```python
from build123d import *

# Parameters (mm, degrees)
SKETCH1_R           = 2.794
BOSS_EXTRUDE1_DEPTH = 2.54
SKETCH2_R           = 3.556
BOSS_EXTRUDE2_DEPTH = 6.35
SKETCH3_R           = 1.397
CUT_EXTRUDE1_DEPTH  = 9.89
SKETCH4_R           = 2.413
CUT_EXTRUDE2_DEPTH  = 0.508
SKETCH5_R           = 1.9939
CUT_EXTRUDE3_DEPTH  = 5.08
CHAMFER1_SIZE       = 0.508
CHAMFER2_SIZE       = 0.254
CHAMFER3_SIZE       = 0.508


with BuildPart() as part:
    # Sketch1 → Boss-Extrude1 (new body)
    with BuildSketch(Plane(origin=(0, 0, 0), x_dir=(1, 0, 0), z_dir=(0, 1, 0))):
        with Locations(Location((0, 0, 0), (0, 0, 270))):  # turned: the seam where the file's is
            Circle(SKETCH1_R)
    extrude(amount=BOSS_EXTRUDE1_DEPTH)

    # Sketch2 → Boss-Extrude2 (add)
    with BuildSketch(Plane(origin=(0, 2.54, 0), x_dir=(1, 0, 0), z_dir=(0, 1, 0))):
        with Locations(Location((0, 0, 0), (0, 0, 270))):  # turned: the seam where the file's is
            Circle(SKETCH2_R)
    extrude(amount=BOSS_EXTRUDE2_DEPTH)

    # Sketch3 → Cut-Extrude1 (cut, through all)
    with BuildSketch(Plane(origin=(0, 8.89, 0), x_dir=(1, 0, 0), z_dir=(0, 1, 0))):
        with Locations(Location((0, 0, 0), (0, 0, 270))):  # turned: the seam where the file's is
            Circle(SKETCH3_R)
    extrude(amount=-CUT_EXTRUDE1_DEPTH, mode=Mode.SUBTRACT)

    # Sketch4 → Cut-Extrude2 (cut)
    with BuildSketch(Plane(origin=(0, 8.89, 0), x_dir=(1, 0, 0), z_dir=(0, 1, 0))):
        with Locations(Location((0, 0, 0), (0, 0, 270))):  # turned: the seam where the file's is
            Circle(SKETCH4_R)
    extrude(amount=-CUT_EXTRUDE2_DEPTH, mode=Mode.SUBTRACT)

    # Sketch5 → Cut-Extrude3 (cut)
    with BuildSketch(Plane.XZ):
        with Locations(Location((0, 0, 0), (0, 0, 270))):  # turned: the seam where the file's is
            Circle(SKETCH5_R)
    extrude(amount=-CUT_EXTRUDE3_DEPTH, mode=Mode.SUBTRACT)

    # Chamfer1
    chamfer1_edges = [part.edges().sort_by_distance(p)[0] for p in [
        (0, 0, -2.794),
        (0, 2.54, -3.556),
        (0, 8.89, -3.556),
    ]]
    chamfer(chamfer1_edges, length=CHAMFER1_SIZE)

    # Chamfer2
    chamfer2_edges = [part.edges().sort_by_distance(p)[0] for p in [
        (0, 0, 1.9939),
    ]]
    chamfer(chamfer2_edges, length=CHAMFER2_SIZE)

    # Chamfer3
    chamfer3_edges = [part.edges().sort_by_distance(p)[0] for p in [
        (0, 8.382, -1.397),
    ]]
    chamfer(chamfer3_edges, length=CHAMFER3_SIZE)


solid = part.part
```
Work out the finished part from the listing and answer in its coordinate system (mm). A direction names the side the tool comes from. Give positions to 0.01 mm unless a question says otherwise; leave off trailing zeros. Loops run counter-clockwise (first coordinate to the right, second up) from the corner with the lowest first, then second, coordinate; pieces in that order, holes last. Notation, with made-up numbers: M 35,23.25 L 94,23.25 A16 ccw 94,42.25 Z; hole C 35.25,-21 d7. An arc over 180 degrees is marked long. One line per item, written item: value. Start each with the question number.
1. Find section C-C (y = 6). Give the vertices of the cut face in (x, z), and give its area (3 significant figures).
2. Find section D-D (y = 8). Give the vertices of the cut face in (x, z), and give its area (3 significant figures).
3. Each of these flat-tipped pins is pushed along its axis until it touches: P1, Ø3, axis at x = 0, z = 0, coming from the -Y side; P2, Ø4, axis at x = -1.5, y = 6, coming from the +Z side; P3, Ø2, axis at y = 5.5, z = -2, coming from the +X side; P4, Ø1.5, axis at y = 8, z = 1.5, coming from the +X side. Where does it stop, or does it pass through?
4. Which of the six approach directions +Z, -Z, +X, -X, +Y, -Y give full straight-line access (tool end or side, diameter ignored) to faces 1 (the face through (-2.728, 1.51, -0.606)), 2 (the face through (-1.364, 6.497, -0.303)), 3 (the face through (1, 8.382, 2))?
5. Find the intervals of material crossed by probe 1 along X at (y, z) = (6.25, 0); probe 2 along X at (y, z) = (3.25, 0); probe 3 along Z at (x, y) = (1, 5.25), in increasing order.
6. Determine the mould class of faces 4 (the face through (-1.468, 8.64, -1.915)), 5 (the face through (-3.47, 5.68, -0.77)) for opening direction Z: released by +Z, released by -Z, zero draft, split by the parting line, or undercut.
Reported:
1. outline: C 0,0 d7.11; hole C 0,0 d2.79
1. area: 33.6 mm²
2. outline: C 0,0 d7.11; hole C 0,0 d3.05
2. area: 32.4 mm²
3. P1: stops at y = 5.08
3. P2: stops at z = 3.56
3. P3: stops at x = 3.41
3. P4: stops at x = 3.48
4. face 1: -Y
4. face 2: +Y, -Y
4. face 3: +Y
5. probe 1: x = -3.56 to -1.4, 1.4 to 3.56
5. probe 2: x = -3.56 to -1.99, 1.99 to 3.56
5. probe 3: z = -3.41 to -0.98, 0.98 to 3.41
6. face 4: undercut
6. face 5: split by the parting line
